Autodesk Inventor part; units mm, degrees
ref_plane "YZ Plane" through (0, 0, 0) normal (1, 0, 0) x (0, 1, 0)
ref_plane "XZ Plane" through (0, 0, 0) normal (0, 1, 0) x (-1, 0, 0)
ref_plane "XY Plane" through (0, 0, 0) normal (0, 0, 1) x (1, 0, 0)
sketch "Sketch1" plane through (0, 0, 0) normal (0, 0, 1) x (1, 0, 0)
  line L0 (-490, 53) -> (490, 53)
  line L1 (490, 53) -> (490, 0)
  line L2 (490, 0) -> (-490, 0)
  line L3 (-490, 0) -> (-490, 53)
  point P0 (0, 0)
  point P1 (0, 0)
  dimension "d0" = 980
  dimension "d1" = 53
extrude "Plate1" add sketch "Sketch1" along normal blind 2
sketch "Sketch2" plane through (490, -2, 0) normal (0, 1, 0) x (-1, 0, 0)
  line L0 (980, 0) -> (0, 0)
  line L1 (0, 0) -> (0, 20)
  line L2 (0, 20) -> (980, 20)
  line L3 (980, 20) -> (980, 0)
edge flange "Flange1" height 20 angle 90 thickness 2 bend radius 2.75 thickness toward (0, 1, 0) relief round relief width 2 relief depth 1 edges at (0, 0, 2) wall of the first edge with corners at (-490, -2, 0) (490, -2, 0) (490, -2, 20) (-490, -2, 20)
bend "Bend1"
corner "Corner1"
sketch "Sketch5" plane through (0, 0, 0) normal (0, 0, -1) x (-1, 0, 0)
  line L0 (490, 53) -> (-490, 53)
  line L1 (490, -2) -> (-490, -2)
  circle A0 centre (0, 53) radius 17.5
  line L2 (243.4, 53) -> (246.6, 53)
  line L3 (246.6, 53) -> (246.6, 26)
  line L4 (246.6, 26) -> (243.4, 26)
  line L5 (243.4, 26) -> (243.4, 53)
  line L6 (-243.4, 53) -> (-246.6, 53)
  line L7 (-246.6, 53) -> (-246.6, 26)
  line L8 (-246.6, 26) -> (-243.4, 26)
  line L9 (-243.4, 26) -> (-243.4, 53)
  line L10 (0, 53) -> (0, -2) construction
  point P0 (0, 0)
  point P1 (-490, -2)
  point P2 (245, 26)
  point P3 (-245, 26)
  point P4 (246.6, 53)
  point P5 (-17.5, 53)
  point P6 (17.5, 53)
  point P7 (-246.6, 53)
  dimension "d45" = 35
  dimension "d48" = 3.2
  dimension "d49" = 490
  dimension "d51" = 28
  dimension "d52" = 27
extrude "Extrusion1" cut sketch "Sketch5" against normal through all contours L3 L4 L5 L0 | L9 L8 L7 L0 | A0 L0 picked at (-2.238, 46.1497)
sketch "Sketch9" plane through (0, 0, 2) normal (0, 0, 1) x (1, 0, 0)
  line L0 (485.6141, 29.596) -> (485.6141, 17.596) construction
  line L1 (485.6141, 17.596) -> (285.6141, 17.596) construction
  line L2 (285.6141, 17.596) -> (285.6141, 29.596) construction
  line L3 (285.6141, 29.596) -> (485.6141, 29.596) construction
  line L4 (-490, 53) -> (490, 53)
  point P0 (0, 0)
  point P1 (1.05, 68)
  point P2 (490, 53)
  dimension "d40" = 200
  dimension "d41" = 12
mark "Mark2"
equation "\"d2\" = Thickness"
equation "\"d3\" = BendReliefWidth"
equation "\"d4\" = BendReliefDepth"
equation "\"d5\" = MinimumRemnant"
equation "\"d6\" = TransitionRadius"
equation "\"d9\" = BendRadius"
equation "\"d10\" = CornerReliefSize"
equation "\"d11\" = GapSize"
equation "\"d12\" = JacobiRadiusSize"
equation "\"BendReliefWidth\" = Thickness"
equation "\"BendReliefDepth\" = 0.5 * Thickness"
equation "\"CornerReliefSize\" = 4 * Thickness"
equation "\"MinimumRemnant\" = 2 * Thickness"
equation "\"TransitionRadius\" = BendRadius"
equation "\"JacobiRadiusSize\" = BendRadius"
equation "\"GapSize\" = Thickness"
properties part number "MSC 343 stringer BOARD  ###" material "Stainless Steel"
CAD build for the part. Positions are in the model's coordinates, mm. A direction names the side the tool comes from. Coordinates: 2 decimals unless noted, no trailing zeros. Loops run counter-clockwise (first coordinate to the right, second up) from the corner with the lowest first, then second, coordinate; pieces in that order, holes last. Notation, with made-up numbers: (-24, 40) - (-3, 40) arc R8 ccw to (-3, 50) - close; hole circle Ø1 at (8.5, 37). An arc over 180 degrees is marked (long way). Use CSV: the item, a comma, the result in double quotes. Start each with the question number.
Q1. Drop flat-ended pins along their axis: P1, Ø15, axis at x = -140, y = 35, coming from the +Z side; P2, Ø2, axis at x = 244.5, z = 0.5, coming from the +Y side; P3, Ø12, axis at x = 142.5, z = 13.5, coming from the +Y side. Give the stop position or say it passes through.
Q2. Probe probe 1 along Y at (x, z) = (-112, 12.25); probe 2 along Z at (x, y) = (-6.5, 20); probe 3 along Y at (x, z) = (-83, 3). List the from-to ranges inside material, lowest first. Write a range as from..to.
Q3. Cut at A-A, the plane x = -45.5. List the corners of the cut face in (y, z).
Q4. Cut at B-B, the plane z = 10.25. List the corners of the cut face in (x, y), then the cut area to 3 significant figures.
Q5. 3-axis set-ups, long thin cutter, end or side, ignore diameter. For faces 1 (the flat face through (-7, 28, 2)), 2 (the cylindrical face through (0.385, 35.504, 0.986)): which of +Z, -Z, +X, -X, +Y, -Y reach the whole face in a straight line?
Here are the results:
1,P1,"z = 2"
1,P2,"y = 26"
1,P3,"y = 0"
2,probe 1,"-2..0"
2,probe 2,"0..2"
2,probe 3,"-1.67..0.63"
3,outline,"(-2, 4.75) arc R4.75 ccw to (2.75, 0) - (53, 0) - (53, 2) - (2.75, 2) arc R2.75 cw to (0, 4.75) - (0, 20) - (-2, 20) - close"
4,outline,"(-490, -2) - (490, -2) - (490, 0) - (-490, 0) - close"
4,area,"1,960 mm2"
5,face 1,"+Z, +X, -X, +Y"
5,face 2,"+Z, -Z, +Y"
